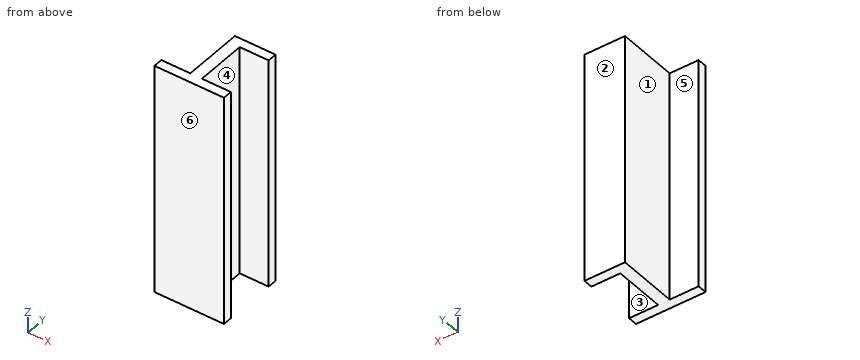
from build123d import *

# Parameters (mm, degrees)
SKETCH_1_W      = 25
SKETCH_1_H      = 8
SKETCH_1_W_2    = 5
EXTRUDE_1_DEPTH = 100


with BuildPart() as part:
    # Эскиз1 → Бобышка-Вытянуть1 (new, symmetric)
    with BuildSketch(Plane.XY):
        with Locations((17.5, -26)):
            Rectangle(SKETCH_1_W, SKETCH_1_H)
        with Locations((2.5, -26)):
            Rectangle(SKETCH_1_W_2, SKETCH_1_H)
        with Locations((-2.5, -26)):
            Rectangle(SKETCH_1_W_2, SKETCH_1_H)
        with Locations((-17.5, -26)):
            Rectangle(SKETCH_1_W, SKETCH_1_H)
        Polygon((0, -22), (5, -22), (5, 22), (0, 22), (0, 30), (-5, 30), (-5, -22), align=None)
        with Locations((17.5, 26)):
            Rectangle(SKETCH_1_W, SKETCH_1_H)
        with Locations((2.5, 26)):
            Rectangle(SKETCH_1_W_2, SKETCH_1_H)
    extrude(amount=EXTRUDE_1_DEPTH, both=True)


solid = part.part
Read the model definition and answer for the solid it produces. Units are mm, in the model's axes. Face numbers are marked on the shaded views. A direction names the side the tool comes from. Give positions to 0.01 mm unless a question says otherwise; leave off trailing zeros. Write each loop counter-clockwise with the first axis right and the second up, starting at its lowest first coordinate (ties: lowest second). Pieces come first, ordered by that corner, then holes. Notation, with made-up numbers: M 46.25,18 L 105.25,18 A9 ccw 105.25,30 Z; hole C 47,23 d5. An arc over 180 degrees is marked long. One line per item, written item: value. Start each with the question number.
(1) Find section C-C (y = -19). Determine the outline of the cut face in (x, z).
(2) Flat-ended cylindrical pins translate along their axes: pin 1 Ø1 at (y, z) = (9.5, -31.5) entering from +X; pin 2 Ø4 at (y, z) = (-19.5, -64.5) entering from -X; pin 3 Ø12.5 at (x, z) = (-15.5, -15.5) entering from +Y. Find the tip coordinate at first contact, or state that the pin passes through.
(3) Find section B-B (z = -22). Determine the outline of the cut face in (x, y).
(4) Find the intervals of material crossed by line 1 (Y direction, x = 8.5, z = 78.5); line 2 (Y direction, x = -7, z = 84.5); line 3 (X direction, y = -1, z = -31.5), in increasing order.
(5) A tool of negligible diameter and unlimited length cuts with its end or side. For the marked faces 4, 5 and 6, from which of +Z, -Z, +X, -X, +Y, -Y can it reach the whole face along a straight path? Write none if from no direction.
(6) Find section D-D (x = -12.5). Determine the outline of the cut face in (y, z), plus the area to 3 significant figures.
(7) Determine the mould class of the marked faces 1, 2 and 3 for opening direction Y: pulls with the +Y half, pulls with the -Y half, needs draft (parallel to the pull), parting line crosses it, or undercut.
(8) Find section A-A (x = 20.5). Determine the outline of the cut face in (y, z).
Results below:
1. outline: M -5,-100 L 5,-100 L 5,100 L -5,100 Z
2. pin 1: stops at x = 5
2. pin 2: stops at x = -5
2. pin 3: stops at y = -22
3. outline: M -30,-30 L 30,-30 L 30,-22 L 5,-22 L 5,22 L 30,22 L 30,30 L -5,30 L -5,-22 L -30,-22 Z
4. line 1: y = -30 to -22, 22 to 30
4. line 2: y = -30 to -22
4. line 3: x = -5 to 5
5. face 4: +Z, -Z, +X
5. face 5: +Z, -Z, -X, +Y
5. face 6: +Z, -Z, +X, -X, -Y
6. outline: M -30,-100 L -22,-100 L -22,100 L -30,100 Z
6. area: 1,600 mm^2
7. face 1: needs draft
7. face 2: pulls with the +Y half
7. face 3: undercut
8. outline: M -30,-100 L -22,-100 L -22,100 L -30,100 Z; M 22,-100 L 30,-100 L 30,100 L 22,100 Z
